Check sheet for the modelled part. Datum: model origin and axes. Units: mm. A direction names the side the tool comes from. Give positions to 0.01 mm unless a question says otherwise; leave off trailing zeros. Loops run counter-clockwise (first coordinate to the right, second up) from the corner with the lowest first, then second, coordinate; pieces in that order, holes last. Notation, with made-up numbers: (-39.75, -38.75) -> (-29.75, -38.75) arc R5 ccw to (-29.75, -31.75) -> close; hole circle Ø10 at (-2.75, 1). An arc over 180 degrees is marked (long way). Write each question's results on one line, items separated by ' | '. Start each with the question number.
1. Cross-section at D-D on y = 12. Record the boundary of the cut face in (x, z), and give its area (3 significant figures).
2. Tool access check on faces 1 (the face through (3.65, 12.696, -37.815)), 2 (the face through (3, 18, -22.84)), 3 (the face through (3.65, 12.696, -0.285)). Record the directions out of +Z, -Z, +X, -X, +Y, -Y that give a thin tool (end or side, any length) a straight path to the whole face; none if there is none.
3. Cross-section at C-C on x = 3. Count the separate pieces of the cut face and the enclosed holes in it, and give its area (3 significant figures).
4. Gauge pin test, flat ends, axial feed: pin 1 Ø4 at (y, z) = (19.4, -6) entering from +X; pin 2 Ø1 at (x, y) = (2.5, 10) entering from -Z. Record the tip position at first contact, or that the pin passes through.
5. Cross-section at A-A on y = 19.4. Record the boundary of the cut face in (x, z).
6. Cross-section at B-B on z = -32.1. Record the boundary of the cut face in (x, y) (3 decimals).
7. Mould release check, pull along Z, two halves, no side actions. Record for faces 4 (the face through (6.6, 25.2, -24.2)), 5 (the face through (7, 0, -19)), 6 (the face through (6.6, 11.4, -37.9)): +Z half, -Z half, draft (parallel to the pull), parting line (faces both ways), or undercut.
8. Material ranges on L1, parallel to Z at x = 2, y = 23; L2, parallel to Y at x = 1.75, z = -9.5 (3 decimals); L3, parallel to Y at x = 7, z = -32.1, recorded low to high. Write a range as from..to.
from build123d import *

# Parameters (mm, degrees)
SKETCH1_W           = 12.5
SKETCH1_H           = 13.005
SKETCH1_R           = 1.65
BOSS_EXTRUDE2_DEPTH = 15
CUT_EXTRUDE1_DEPTH  = 6.2
FILLET1_R           = 1


with BuildPart() as part:
    # Sketch1 → Boss-Extrude2 (new body)
    # profile 1 of 5: a face of its own
    with BuildSketch(Plane(origin=(0, 0, 0), x_dir=(0, 0, -1), z_dir=(1, 0, 0))):
        with Locations((6.25, 18.8975)):
            Rectangle(SKETCH1_W, SKETCH1_H)
        with Locations((6, 19.4)):
            Circle(SKETCH1_R, mode=Mode.SUBTRACT)
    # profile 2 of 5: a face of its own
    with BuildSketch(Plane(origin=(0, 0, 0), x_dir=(0, 0, -1), z_dir=(1, 0, 0))):
        Polygon((12.5, 12.395), (0, 12.395), (0, 10.325), (15.26, 10.325), (15.26, 25.4), (12.5, 25.4), align=None)
    # profile 3 of 5: a face of its own
    with BuildSketch(Plane(origin=(0, 0, 0), x_dir=(0, 0, -1), z_dir=(1, 0, 0))):
        Polygon((15.26, 10.325), (0, 10.325), (0, 0), (38.1, 0), (38.1, 10.325), (22.84, 10.325), (22.84, 25.4), (15.26, 25.4), align=None)
        with Locations((19.05, 5.1625)):
            Circle(SKETCH1_R, mode=Mode.SUBTRACT)
    # profile 4 of 5: a face of its own
    with BuildSketch(Plane(origin=(0, 0, 0), x_dir=(0, 0, -1), z_dir=(1, 0, 0))):
        Polygon((25.6, 25.4), (22.84, 25.4), (22.84, 10.325), (38.1, 10.325), (38.1, 12.395), (25.6, 12.395), align=None)
    # profile 5 of 5: a face of its own
    with BuildSketch(Plane(origin=(0, 0, 0), x_dir=(0, 0, -1), z_dir=(1, 0, 0))):
        with Locations((31.85, 18.8975)):
            Rectangle(SKETCH1_W, SKETCH1_H)
        with Locations((32.1, 19.4)):
            Circle(SKETCH1_R, mode=Mode.SUBTRACT)
    extrude(amount=BOSS_EXTRUDE2_DEPTH)

    # Sketch1_9 → Cut-Extrude1 (cut)
    with BuildSketch(Plane(origin=(0, 0, 0), x_dir=(0, 0, -1), z_dir=(1, 0, 0))):
        Polygon((22.84, 10.325), (38.1, 10.325), (38.1, 12.395), (25.6, 12.395), (25.6, 25.4), (22.84, 25.4), align=None)
        Polygon((15.26, 25.4), (15.26, 10.325), (0, 10.325), (0, 12.395), (12.5, 12.395), (12.5, 25.4), align=None)
    extrude(amount=CUT_EXTRUDE1_DEPTH, mode=Mode.SUBTRACT)

    # Fillet1
    fillet1_edges = [part.edges().sort_by_distance(p)[0] for p in [
        (3.1, 10.325, -22.84),
        (3.1, 10.325, -38.1),
        (3.1, 12.395, -38.1),
        (3.1, 12.395, -25.6),
        (3.1, 25.4, -25.6),
        (3.1, 25.4, -22.84),
        (6.2, 11.36, -38.1),
        (6.2, 25.4, -24.22),
        (6.2, 25.4, -13.88),
        (3.1, 25.4, -15.26),
        (3.1, 25.4, -12.5),
        (3.1, 12.395, -12.5),
        (6.2, 11.36, 0),
        (3.1, 12.395, 0),
        (3.1, 10.325, 0),
        (3.1, 10.325, -15.26),
    ]]
    fillet(fillet1_edges, radius=FILLET1_R)


solid = part.part
Geometry says:
1) outline: (0, -22.84) -> (6.2, -22.84) -> (6.2, -37.1) arc R1 ccw to (7.2, -38.1) -> (15, -38.1) -> (15, 0) -> (7.2, 0) arc R1 ccw to (6.2, -1) -> (6.2, -15.26) -> (0, -15.26) -> close | area: 382 mm^2
2) face 1: -Z, -X | face 2: -X, +Y | face 3: +Z, -X
3) separate pieces: 3 | enclosed holes: 3 | area: 805 mm^2
4) pin 1: x = 15 | pin 2: z = -38.08
5) outline: (0, -38.1) -> (15, -38.1) -> (15, -33.75) -> (0, -33.75) -> close; (0, -30.45) -> (15, -30.45) -> (15, -7.65) -> (0, -7.65) -> (0, -12.5) -> (6.2, -12.5) -> (6.2, -15.26) -> (0, -15.26) -> (0, -22.84) -> (6.2, -22.84) -> (6.2, -25.6) -> (0, -25.6) -> close; (0, -4.35) -> (15, -4.35) -> (15, 0) -> (0, 0) -> close
6) outline: (0, 0) -> (15, 0) -> (15, 17.75) -> (0, 17.75) -> (0, 12.395) -> (6.2, 12.395) -> (6.2, 10.325) -> (0, 10.325) -> close; (0, 21.05) -> (15, 21.05) -> (15, 25.4) -> (0, 25.4) -> close
7) face 4: undercut | face 5: draft | face 6: -Z half
8) L1: -38.1..-25.6, -22.84..-15.26, -12.5..0 | L2: 0..10.325, 12.395..25.4 | L3: 0..17.75, 21.05..25.4
